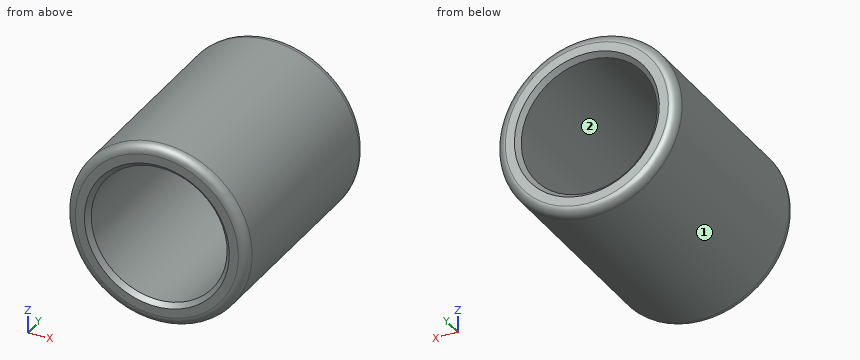
from build123d import *

# Parameters (mm, degrees)
ESBO_O1_R                = 20
ESBO_O1_R_2              = 15
RESSALTO_EXTRUS_O1_DEPTH = 50
FILETE1_R                = 2
CHANFRO1_SIZE            = 1


with BuildPart() as part:
    # Esboço1 → Ressalto-extrusão1 (new body)
    with BuildSketch(Plane(origin=(0, 0, 0), x_dir=(1, 0, 0), z_dir=(0, 1, 0))):
        with Locations(Location((0, 0, 0), (0, 0, 270))):  # turned: the seam where the file's is
            Circle(ESBO_O1_R)
        with Locations(Location((0, 0, 0), (0, 0, 270))):  # turned: the seam where the file's is
            Circle(ESBO_O1_R_2, mode=Mode.SUBTRACT)
    extrude(amount=RESSALTO_EXTRUS_O1_DEPTH)

    # Filete1
    filete1_edges = [part.edges().sort_by_distance(p)[0] for p in [
        (0, 0, -20),
        (0, 50, -20),
    ]]
    fillet(filete1_edges, radius=FILETE1_R)

    # Chanfro1
    chanfro1_edges = [part.edges().sort_by_distance(p)[0] for p in [
        (0, 0, -15),
        (0, 50, -15),
    ]]
    chamfer(chanfro1_edges, length=CHANFRO1_SIZE)


solid = part.part
Geometry: final body of the model. Coordinates: model frame, mm. Face numbers are marked on the shaded views. Give positions to 0.01 mm unless a question says otherwise; leave off trailing zeros. Loops run counter-clockwise (first coordinate to the right, second up) from the corner with the lowest first, then second, coordinate; pieces in that order, holes last. Notation, with made-up numbers: (76.25, -25.5) -> (131.25, -25.5) arc R10 ccw to (131.25, -18.5) -> close; hole circle Ø5 at (23, -30.75). An arc over 180 degrees is marked (long way). Put each result on its own line as item: value.
1. Pull-direction query (Z, two-part tool) for the marked faces 1 and 2; classes: released by +Z, released by -Z, zero draft, split by the parting line, or undercut.
Taken from the geometry:
face 1: split by the parting line
face 2: undercut
2. Cut plane B-B (z = 0). Return the cut outline in (x, y), plus the area to 3 significant figures.
Taken from the geometry:
outline: (-20, 2) arc R2 ccw to (-18, 0) -> (-16, 0) -> (-15, 1) -> (-15, 49) -> (-16, 50) -> (-18, 50) arc R2 ccw to (-20, 48) -> close; (15, 1) -> (16, 0) -> (18, 0) arc R2 ccw to (20, 2) -> (20, 48) arc R2 ccw to (18, 50) -> (16, 50) -> (15, 49) -> close
area: 495 mm2
3. Ray query, line 1 along X through (y, z) = (32.5, 0); line 2 along Z through (x, y) = (-0.5, 30); line 3 along X through (y, z) = (31.5, -9.5). Return the intervals inside material, ascending. Write a range as [from, to].
Taken from the geometry:
line 1: x = [-20, -15], [15, 20]
line 2: z = [-19.99, -14.99], [14.99, 19.99]
line 3: x = [-17.6, -11.61], [11.61, 17.6]
4. Pin query (flat end, axial travel): P1, Ø10, axis at x = -15, y = 31.5, coming from the +Z side; P2, Ø5, axis at y = 37.5, z = 14.5, coming from the -X side; P3, Ø1, axis at x = 12, y = 6.5, coming from the +Z side. Return the tip coordinate at first contact, or that it passes through.
Taken from the geometry:
P1: stops at z = 17.32
P2: stops at x = -16
P3: stops at z = 16.36
5. Cut plane A-A (x = 0). Return the cut outline in (y, z), plus the area to 3 significant figures.
Taken from the geometry:
outline: (0, -18) arc R2 ccw to (2, -20) -> (48, -20) arc R2 ccw to (50, -18) -> (50, -16) -> (49, -15) -> (1, -15) -> (0, -16) -> close; (0, 16) -> (1, 15) -> (49, 15) -> (50, 16) -> (50, 18) arc R2 ccw to (48, 20) -> (2, 20) arc R2 ccw to (0, 18) -> close
area: 495 mm2
6. Cut plane C-C (y = 43.5). Return the cut outline in (x, z).
Taken from the geometry:
outline: circle Ø40 at (0, 0); hole circle Ø30 at (0, 0)
